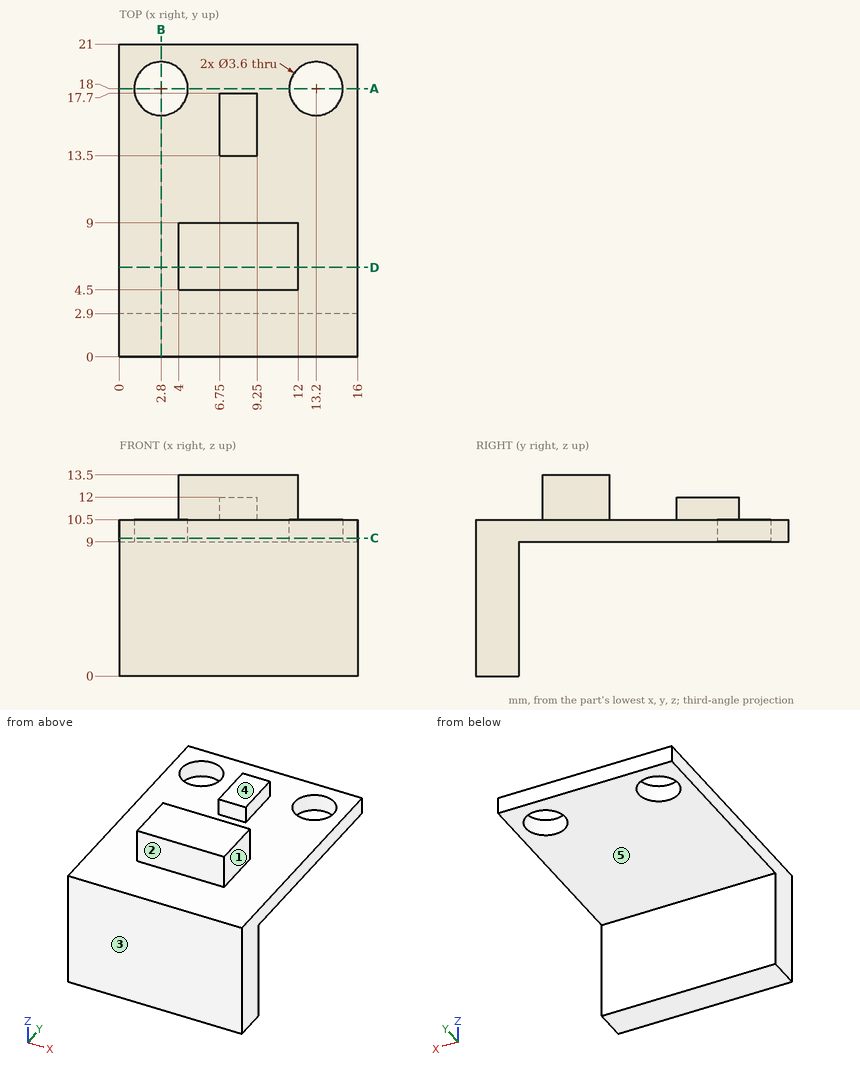
Job drawing, mm, ordinate dimensions from the low corner. One solid piece. A direction names the side the tool comes from. Coordinates: 2 decimals unless noted, no trailing zeros. Loops run counter-clockwise (first coordinate to the right, second up) from the corner with the lowest first, then second, coordinate; pieces in that order, holes last. Notation, with made-up numbers: (69.5, -24.5) -> (83.5, -24.5) arc R14 cw to (83.5, -0.5) -> close; hole circle Ø7 at (18, 52). An arc over 180 degrees is marked (long way). One line per item, written item: value.
1. Slice it at A-A on y = 18. Write the cut outline in (x, z), and give its area (3 significant figures).
Answers:
outline: (0, 9) -> (1, 9) -> (1, 10.5) -> (0, 10.5) -> close; (4.6, 9) -> (11.4, 9) -> (11.4, 10.5) -> (4.6, 10.5) -> close; (15, 9) -> (16, 9) -> (16, 10.5) -> (15, 10.5) -> close
area: 13.2 mm^2
2. Drill centre lines: line 1 (Y direction, x = 13.2, z = 9.55); line 2 (Z direction, x = 7.75, y = 15.5); line 3 (Y direction, x = 6.75, z = 3). Where is each one in solid material? Low to high. Write a range as [from, to].
Answers:
line 1: y = [0, 16.2], [19.8, 21]
line 2: z = [9, 12]
line 3: y = [0, 2.9]
3. Slice it at D-D on y = 6. Write the cut outline in (x, z).
Answers:
outline: (0, 9) -> (16, 9) -> (16, 10.5) -> (12, 10.5) -> (12, 13.5) -> (4, 13.5) -> (4, 10.5) -> (0, 10.5) -> close
4. Slice it at C-C on z = 9.25. Write the cut outline in (x, y), and give its area (3 significant figures).
Answers:
outline: (0, 0) -> (16, 0) -> (16, 21) -> (0, 21) -> close; hole circle Ø3.6 at (2.8, 18); hole circle Ø3.6 at (13.2, 18)
area: 316 mm^2
5. Slice it at B-B on x = 2.8. Write the cut outline in (y, z).
Answers:
outline: (0, 0) -> (2.9, 0) -> (2.9, 9) -> (16.2, 9) -> (16.2, 10.5) -> (0, 10.5) -> close; (19.8, 9) -> (21, 9) -> (21, 10.5) -> (19.8, 10.5) -> close
6. Which spindle directions (+Z, -Z, +X, -X, +Y, -Y) get a long thin tool onto all of the face, cutting with end or side? Do the marked faces 1, 2, 3, 4 and 5. Say none if no direction does.
Answers:
face 1: +Z, +X, +Y, -Y
face 2: +Z, +X, -X, -Y
face 3: +Z, -Z, +X, -X, -Y
face 4: +Z, +X, -X, +Y
face 5: -Z, +X, -X, +Y
7. Flat gauge pins, fed straight in: P1, Ø2.5, axis at x = 9.5, z = 12.5, coming from the -Y side; P2, Ø4.5, axis at x = 6, z = 6, coming from the +Y side; P3, Ø1.2, axis at x = 7.5, y = 16, coming from the +Z side. Where does each tip first touch, or does it go through?
Answers:
P1: stops at y = 4.5
P2: stops at y = 2.9
P3: stops at z = 12
